Part print with two shaded views. Sizes in mm from the minimum x, y, z corner. A direction names the side the tool comes from. Give positions to 0.01 mm unless a question says otherwise; leave off trailing zeros. Order: outer loops, then holes, each group sorted by start corner. A loop starts at its lowest first (then second) coordinate and runs counter-clockwise, first axis right, second up. Notation, with made-up numbers: (12, 31) -> (65, 31) arc R29 ccw to (65, 52) -> close; hole circle Ø1 at (-4, 16.5). An arc over 180 degrees is marked (long way). Write item = value, one per line. Start each with the question number.
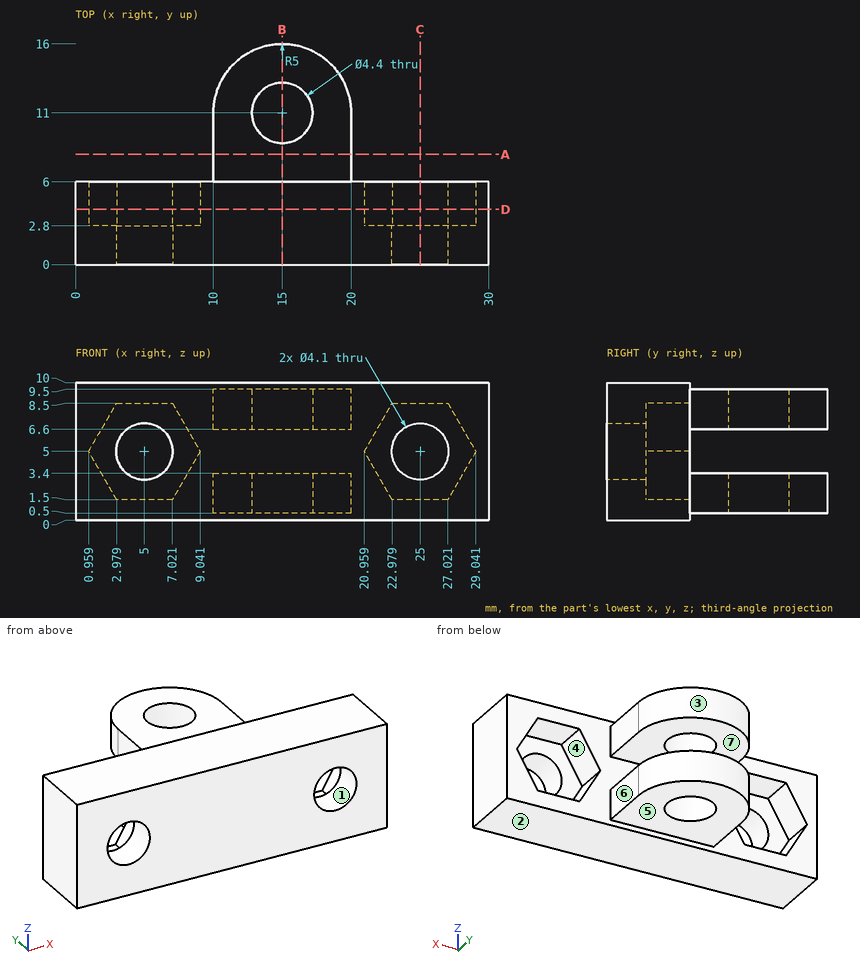
(1) Cut at C-C, the plane x = 25. Give the cut face in (y, z).
(2) Cut at A-A, the plane y = 8. Give the cut face in (x, z).
(3) 3-axis set-ups, long thin cutter, end or side, ignore diameter. For the marked faces 4, 5, 6 and 7: which of +Z, -Z, +X, -X, +Y, -Y reach the whole face in a straight line?
(4) Cut at B-B, the plane x = 15. Give the cut face in (y, z).
(5) Wall check: line 1 (X direction, y = 0.75, z = 5); line 2 (Y direction, x = 15, z = 8.25); line 3 (X direction, y = 11, z = 8.55). Give the ranges that are in metal, low to high. Write a range as [from, to].
(6) Flat gauge pins, fed straight in: P1, Ø4, axis at x = 19.5, y = 11, coming from the -Z side; P2, Ø5, axis at x = 10.5, y = 14, coming from the +Z side; P3, Ø1.5, axis at y = 9, z = 2.5, coming from the +X side; P4, Ø2.5, axis at x = 15, y = 11, coming from the -Z side. Where does each tip first touch, or does it go through?
(7) Mould opens along X. For the marked faces 1, 2 and 3 say: released by +X, released by -X, zero draft, split by the parting line, or undercut.
(8) Cut at D-D, the plane y = 4. Give the cut face in (x, z), plus the area to 3 significant figures.
Results:
q1.outline = (0, 0) -> (6, 0) -> (6, 1.5) -> (2.8, 1.5) -> (2.8, 2.95) -> (0, 2.95) -> close; (0, 7.05) -> (2.8, 7.05) -> (2.8, 8.5) -> (6, 8.5) -> (6, 10) -> (0, 10) -> close
q2.outline = (10, 0.5) -> (20, 0.5) -> (20, 3.4) -> (10, 3.4) -> close; (10, 6.6) -> (20, 6.6) -> (20, 9.5) -> (10, 9.5) -> close
q3.face_4 = +Y
q3.face_5 = -Z, +X, -X, +Y
q3.face_6 = +Z, -Z, +X, +Y
q3.face_7 = +X, -X, +Y
q4.outline = (0, 0) -> (6, 0) -> (6, 0.5) -> (8.8, 0.5) -> (8.8, 3.4) -> (6, 3.4) -> (6, 6.6) -> (8.8, 6.6) -> (8.8, 9.5) -> (6, 9.5) -> (6, 10) -> (0, 10) -> close; (13.2, 0.5) -> (16, 0.5) -> (16, 3.4) -> (13.2, 3.4) -> close; (13.2, 6.6) -> (16, 6.6) -> (16, 9.5) -> (13.2, 9.5) -> close
q5.line_1 = [0, 2.95], [7.05, 22.95], [27.05, 30]
q5.line_2 = [0, 8.8], [13.2, 16]
q5.line_3 = [10, 12.8], [17.2, 20]
q6.P1 = 0.5
q6.P2 = 9.5
q6.P3 = 20
q6.P4 = through
q7.face_1 = undercut
q7.face_2 = zero draft
q7.face_3 = split by the parting line
q8.outline = (0, 0) -> (30, 0) -> (30, 10) -> (0, 10) -> close; hole (0.96, 5) -> (2.98, 1.5) -> (7.02, 1.5) -> (9.04, 5) -> (7.02, 8.5) -> (2.98, 8.5) -> close; hole (20.96, 5) -> (22.98, 1.5) -> (27.02, 1.5) -> (29.04, 5) -> (27.02, 8.5) -> (22.98, 8.5) -> close
q8.area = 215 mm2
